Check sheet for the modelled part. Datum: model origin and axes. Units: mm. Face numbers are marked on the shaded views. Give positions to 0.01 mm unless a question says otherwise; leave off trailing zeros. Order: outer loops, then holes, each group sorted by start corner. A loop starts at its lowest first (then second) coordinate and runs counter-clockwise, first axis right, second up. Notation, with made-up numbers: (-10, 37) - (4, 37) arc R26 cw to (4, 66) - close; hole circle Ø10 at (50, -35). An arc over 180 degrees is marked (long way). Answer in a Markdown table with one row per item.
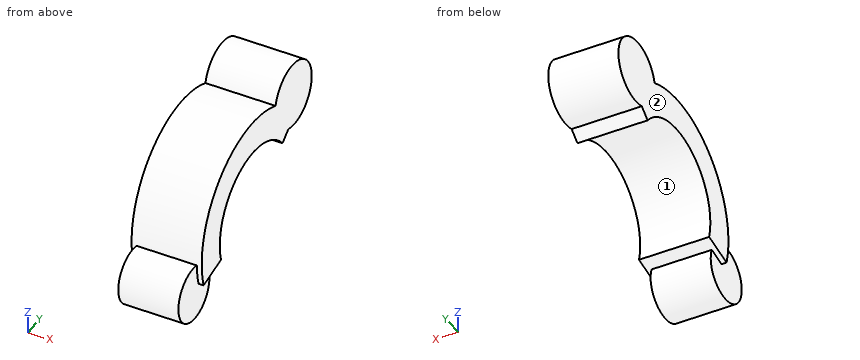
from build123d import *

# Parameters (mm, degrees)
GANCHO_TROCLEAR_DEPTH = 14
SKETCH2_R             = 6.5
OLECRANON_DEPTH       = 14
SKETCH3_R             = 5.5
CORONOIDES_DEPTH      = 12


with BuildPart() as part:
    # Sketch1 → Gancho_troclear (new body)
    with BuildSketch(Plane(origin=(-7, 0, 0), x_dir=(0, 0, -1), z_dir=(1, 0, 0))):
        with BuildLine():
            Line((4.917561857, -18.352590699), (3.261119968, -12.170665411))
            ThreePointArc((3.261119968, -12.170665411), (-11.176336498, -5.818032527), (-8.099123882, 9.652159983))
            Line((-8.099123882, 9.652159983), (-12.212964584, 14.554844419))
            ThreePointArc((-12.212964584, 14.554844419), (-16.85320583, -8.773223651), (4.917561857, -18.352590699))
        make_face()
    extrude(amount=GANCHO_TROCLEAR_DEPTH)

    # Sketch2 → Olecranon (add)
    with BuildSketch(Plane(origin=(-7, 0, 0), x_dir=(0, 0, -1), z_dir=(1, 0, 0))):
        with Locations((-16.086933305, 13.498539803)):
            Circle(SKETCH2_R)
    extrude(amount=OLECRANON_DEPTH)

    # Sketch3 → Coronoides (add)
    with BuildSketch(Plane(origin=(-6, 0, 0), x_dir=(0, 0, -1), z_dir=(1, 0, 0))):
        with Locations((6, -20)):
            Circle(SKETCH3_R)
    extrude(amount=CORONOIDES_DEPTH)


solid = part.part
(1) Cross-section at A-A, the plane z = 12. Record the cut outline in (x, y), then the cut area to 3 significant figures.
Geometry says:
| item | result |
|---|---|
| outline | (-7, -14.73) - (7, -14.73) - (7, -3.84) - (-7, -3.84) - close; (-7, 3.84) - (7, 3.84) - (7, 18.55) - (-7, 18.55) - close |
| area | 358 mm² |
(2) Mould release check, pull along Y, two halves, no side actions. Record for the marked faces 1 and 2: pulls with the +Y half, pulls with the -Y half, needs draft (parallel to the pull), parting line crosses it, or undercut.
Geometry says:
| item | result |
|---|---|
| face 1 | undercut |
| face 2 | needs draft |
(3) Cross-section at B-B, the plane z = 0. Record the cut outline in (x, y), then the cut area to 3 significant figures.
Geometry says:
| item | result |
|---|---|
| outline | (-7, -19) - (7, -19) - (7, -12.6) - (-7, -12.6) - close |
| area | 89.6 mm² |
(4) Cross-section at D-D, the plane x = -1. Record the cut outline in (y, z), then the cut area to 3 significant figures.
Geometry says:
| item | result |
|---|---|
| outline | (-18.99, -0.59) arc R5.5 ccw (long way) to (-14.88, -3.99) - (-12.17, -3.26) arc R12.6 cw to (9.65, 8.1) - (11.72, 9.83) arc R6.5 ccw (long way) to (7.18, 17.59) arc R19 ccw to start |
| area | 460 mm² |
(5) Gauge pin test, flat ends, axial feed: P1, Ø3, axis at x = -0.5, z = 7.5, coming from the -Y side; P2, Ø4, axis at x = -3, y = -6.5, coming from the +Z side; P3, Ø1, axis at x = 1, y = 0.5, coming from the +Z side. Record the tip position at first contact, or that the pin passes through.
Geometry says:
| item | result |
|---|---|
| P1 | y = -18.03 |
| P2 | z = 18.46 |
| P3 | z = 19 |
(6) Thickness scan on L1, parallel to X at y = -20.5, z = -1.5; L2, parallel to Y at x = -1.25, z = 10.5; L3, parallel to Z at x = -1.5, y = -17. Record the ranges inside material, lowest first.
Geometry says:
| item | result |
|---|---|
| L1 | -6 to 6 |
| L2 | -15.84 to -6.96, 6.96 to 16.82 |
| L3 | -10.61 to 8.49 |
(7) Cross-section at C-C, the plane y = -20. Record the cut outline in (x, z), then the cut area to 3 significant figures.
Geometry says:
| item | result |
|---|---|
| outline | (-6, -11.5) - (6, -11.5) - (6, -0.5) - (-6, -0.5) - close |
| area | 132 mm² |
